Study the drawing (mm; zero at the part's minimum x, y, z) and answer. A direction names the side the tool comes from. Give positions to 0.01 mm unless a question says otherwise; leave off trailing zeros. Write each loop counter-clockwise with the first axis right and the second up, starting at its lowest first coordinate (ties: lowest second). Pieces come first, ordered by that corner, then holes. Notation, with made-up numbers: M 50,-25.5 L 63,-25.5 A12 ccw 63,-14.5 Z; hole C 72,-32.5 d2. An arc over 180 degrees is marked long. Use a Markdown table: item, result. Add a question column.
Item 1: A cutting plane is placed at C-C on y = 7. Determine the outline of the cut face in (x, z) (1 decimal), then the cut area to 3 significant figures.
Item 2: A cutting plane is placed at B-B on z = 12.7. Count the separate pieces of the cut face and the enclosed holes in it, then the cut area to 3 significant figures.
Item 3: For the marked faces 5, 6 and 7, determine the directions among +Z, -Z, +X, -X, +Y, -Y from which every point of the face is accessible in a straight line to the end or side of a thin tool.
Item 4: The mould has two halves that part along X. Classify the marked faces 1, 2, 3 and 4: pulls with the +X half, pulls with the -X half, needs draft (parallel to the pull), parting line crosses it, or undercut.
Item 5: Given P1, Ø9, axis at x = 25.4, z = 12.7, coming from the -Y side; P2, Ø8, axis at x = 19.5, y = 48.5, coming from the +Z side; P3, Ø1, axis at y = 11.5, z = 8.5, coming from the -X side (1 decimal), each flat-ended and moving along its own axis, determine where each tip first touches the part or whether it passes through.
Item 6: Consider probe 1 along Z at (x, y) = (25.4, 61.75) (1 decimal); probe 2 along Z at (x, y) = (25, 3); probe 3 along Y at (x, z) = (27, 8). Determine where each line is inside the solid, lowest interval first. Write a range as [from, to].
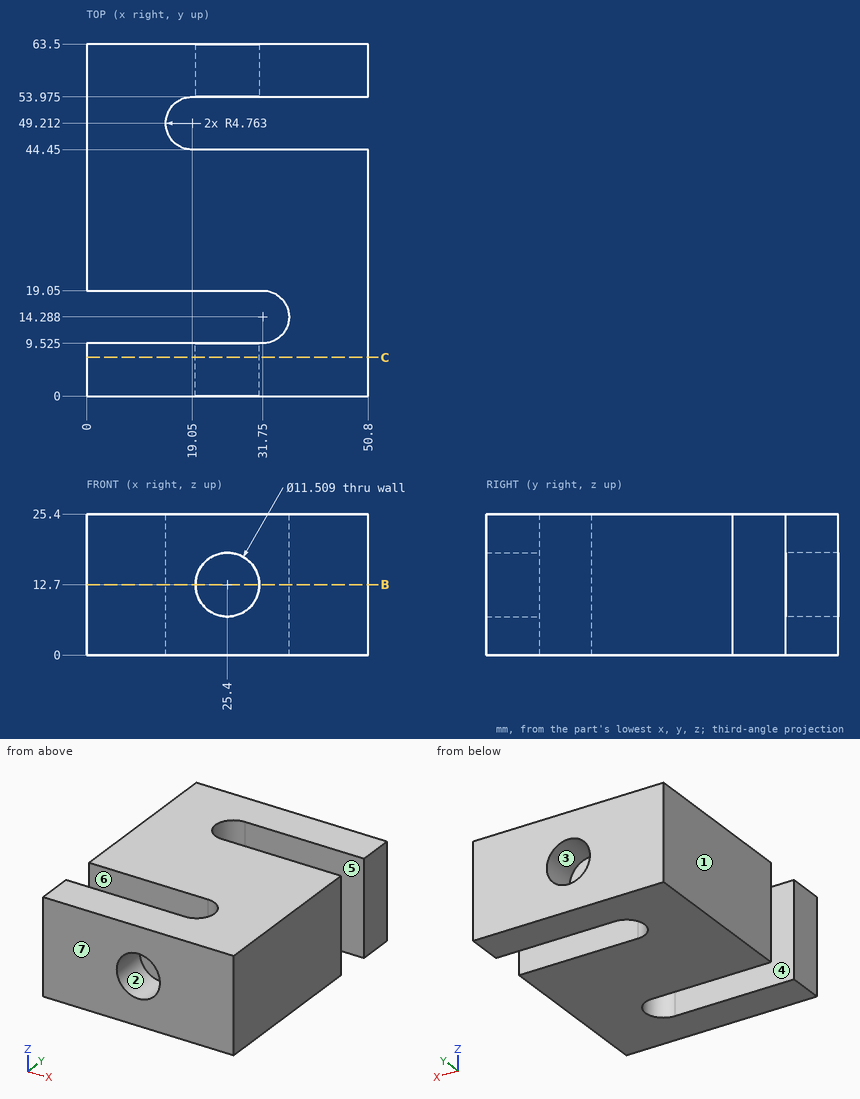
Filled in:
| question | item | result |
|---|---|---|
| 1 | outline | M 0,0 L 50.8,0 L 50.8,25.4 L 0,25.4 Z; hole C 25.4,12.7 d11.5 |
| 1 | area | 1,190 mm² |
| 2 | separate pieces | 3 |
| 2 | enclosed holes | 0 |
| 2 | area | 2,330 mm² |
| 3 | face 5 | +Z, -Z, +X |
| 3 | face 6 | +Z, -Z, -X |
| 3 | face 7 | +Z, -Z, +X, -X, -Y |
| 4 | face 1 | pulls with the -X half |
| 4 | face 2 | undercut |
| 4 | face 3 | undercut |
| 4 | face 4 | needs draft |
| 5 | P1 | y = 19.05 |
| 5 | P2 | through |
| 5 | P3 | x = 35.2 |
| 6 | probe 1 | [0, 6.9], [18.5, 25.4] |
| 6 | probe 2 | [0, 6.96], [18.44, 25.4] |
| 6 | probe 3 | [19.05, 44.45] |
